Design review of the part built by this model. Coordinates are the model's own, in mm. A direction names the side the tool comes from. Coordinates: 2 decimals unless noted, no trailing zeros. Write each loop counter-clockwise with the first axis right and the second up, starting at its lowest first coordinate (ties: lowest second). Pieces come first, ordered by that corner, then holes.
Q1. The part is to be moulded in two halves that separate along Y. For faces 4 (the face through (5, -5, 2.7)), 5 (the face through (2.46, -2.36, 2.86)), say which applies: +Y half, -Y half, draft (parallel to the pull), parting line (faces both ways), or undercut.
Q2. Add section D-D, the plane z = 0.95. Give the boundary of the cut face in (x, y), plus the area to 3 significant figures.
Q3. To check wall thickness, follow probe 1 along Y at (x, z) = (-3.25, 2.65); probe 2 along Y at (x, z) = (4.75, 4.9); probe 3 along Z at (x, y) = (-5.25, -5). State the ranges of each line that lie inside material, in increasing order.
Q4. Clearance check with flat-ended pins moving along their axes: pin 1 Ø2 at (x, y) = (-3.5, -5) entering from -Z; pin 2 Ø0.7 at (x, y) = (0, -5.5) entering from -Z; pin 3 Ø0.7 at (x, y) = (0, -4.5) entering from +Z; pin 4 Ø1.7 at (x, z) = (2, 4) entering from -Y. State where each tip first meets the part, or that it passes through.
Q5. Machinability: for faces 1 (the face through (-5, -5, 3.1)), 2 (the face through (0, 0, 5.8)), 3 (the face through (0, -5, 2.7)), which of the approach directions +Z, -Z, +X, -X, +Y, -Y give a long, thin tool a straight path to every point of the face, cutting with its end or side? Answer none if there is none.
Q6. Add section B-B, the plane y = -1.75. Give the boundary of the cut face in (x, z), plus the area to 3 significant figures.
Q7. Add section A-A, the plane x = 3.25. Give the boundary of the cut face in (y, z), plus the area to 3 significant figures.
Q8. Add section C-C, the plane z = 2.3. Give the boundary of the cut face in (x, y), plus the area to 3 significant figures.
from build123d import *

# Parameters (mm, degrees)
F0_W     = 12.7
F0_H     = 6.5
F0_R     = 1
F1_DEPTH = 5.8
F4_W     = 0.9
F4_H     = 3.5
F5_DEPTH = 0.4
F2_W     = 1.2
F2_H     = 2.9
F6_DEPTH = 0.5
F7_R     = 0.4


with BuildPart() as f1:
    # F0 (on Top) → F1 (new body)
    with BuildSketch(Plane.XY):
        Rectangle(F0_W, F0_H)
        with Locations((-3.25, -1.75)):
            Circle(F0_R, mode=Mode.SUBTRACT)
        with Locations((3.25, -1.75)):
            Circle(F0_R, mode=Mode.SUBTRACT)
    extrude(amount=F1_DEPTH)

    # F4 (on offset) → F5 (join)
    with BuildSketch(Plane.XY.offset(2.7)):
        with Locations((-5.08, -5)):
            Rectangle(F4_W, F4_H)
        with Locations((0, -5)):
            Rectangle(F4_W, F4_H)
        with Locations((5.08, -5)):
            Rectangle(F4_W, F4_H)
    extrude(amount=F5_DEPTH)

    # F2 (on face) → F6 (join)
    with BuildSketch(Plane(origin=(0, 3.25, 0), x_dir=(-1, 0, 0), z_dir=(0, 1, 0))):
        with Locations((1.85, 2.95)):
            Rectangle(F2_W, F2_H)
    extrude(amount=F6_DEPTH)

    # F7
    f7_edges = [f1.edges().sort_by_distance(p)[0] for p in [
        (-2.45, 3.75, 2.95),
        (-1.25, 3.75, 2.95),
    ]]
    fillet(f7_edges, radius=F7_R)


solid = f1.part
Here are the results:
1. face 4: draft
1. face 5: undercut
2. outline: (-6.35, -3.25) - (6.35, -3.25) - (6.35, 3.25) - (-6.35, 3.25) - close; hole circle Ø2 at (-3.25, -1.75); hole circle Ø2 at (3.25, -1.75)
2. area: 76.3 mm2
3. probe 1: y = -3.25 to -2.75, -0.75 to 3.25
3. probe 2: y = -3.25 to 3.25
3. probe 3: z = 2.7 to 3.1
4. pin 1: passes through
4. pin 2: stops at z = 2.7
4. pin 3: stops at z = 3.1
4. pin 4: stops at y = -3.25
5. face 1: +Z, +X, -X, -Y
5. face 2: +Z, +X, -X, +Y, -Y
5. face 3: -Z, +X, -X, -Y
6. outline: (-6.35, 0) - (-4.25, 0) - (-4.25, 5.8) - (-6.35, 5.8) - close; (-2.25, 0) - (2.25, 0) - (2.25, 5.8) - (-2.25, 5.8) - close; (4.25, 0) - (6.35, 0) - (6.35, 5.8) - (4.25, 5.8) - close
6. area: 50.5 mm2
7. outline: (-3.25, 0) - (-2.75, 0) - (-2.75, 5.8) - (-3.25, 5.8) - close; (-0.75, 0) - (3.25, 0) - (3.25, 5.8) - (-0.75, 5.8) - close
7. area: 26.1 mm2
8. outline: (-6.35, -3.25) - (6.35, -3.25) - (6.35, 3.25) - (-1.25, 3.25) - (-1.25, 3.35) arc R0.4 ccw to (-1.65, 3.75) - (-2.05, 3.75) arc R0.4 ccw to (-2.45, 3.35) - (-2.45, 3.25) - (-6.35, 3.25) - close; hole circle Ø2 at (-3.25, -1.75); hole circle Ø2 at (3.25, -1.75)
8. area: 76.8 mm2
